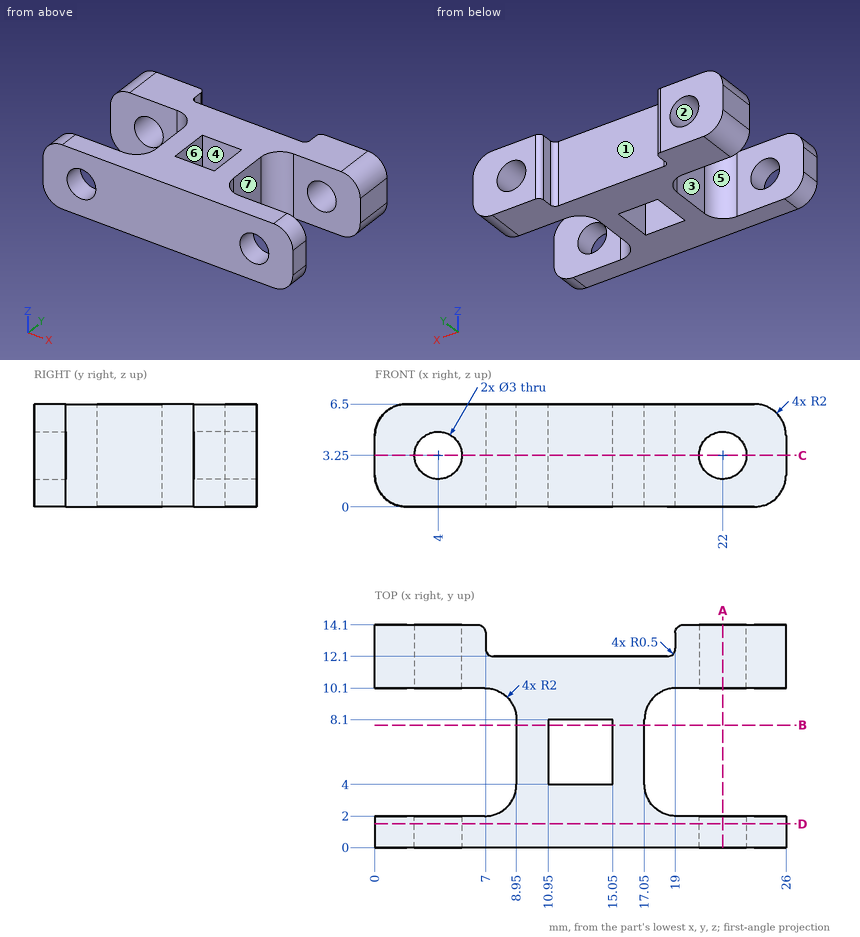
Drawing for the job (mm, zero at the part's lowest x, y, z). A direction names the side the tool comes from. Round coordinates to 2 decimals unless told otherwise and drop trailing zeros. Loops run counter-clockwise (first coordinate to the right, second up) from the corner with the lowest first, then second, coordinate; pieces in that order, holes last. Notation, with made-up numbers: (-7, 89) -> (1, 89) arc R16 ccw to (1, 113) -> close; hole circle Ø5 at (61.25, 64). An arc over 180 degrees is marked (long way). Use one line per item in the form item = value. Start each with the question number.
Item 1: Tool access for the marked faces 5, 6 and 7: list every direction of +Z, -Z, +X, -X, +Y, -Y with a clear straight run to the whole face (end or side of a thin tool).
Item 2: Band-saw the part on D-D (y = 1.5). List the corners of the cut face in (x, z).
Item 3: Two-plate mould, pull along Y, no slides. Class the marked faces 1, 2, 3 and 4: released by +Y, released by -Y, zero draft, split by the parting line, or undercut.
Item 4: Drill centre lines: line 1 along X through (y, z) = (11.1, 3.25); line 2 along Z through (x, y) = (22, 1.5); line 3 along Y through (x, z) = (13, 3.75). Where is each one in solid material? Low to high.
Item 5: Band-saw the part on C-C (z = 3.25). Give the number of separate pieces and of enclosed holes in the cut face, plus the area to 3 significant figures.
Item 6: Band-saw the part on B-B (y = 7.75). List the corners of the cut face in (x, z), plus the area to 3 significant figures.
Item 7: Band-saw the part on A-A (x = 22). List the corners of the cut face in (y, z), plus the area to 3 significant figures.
Item 8: Drop flat-ended pins along their axis: pin 1 Ø1.2 at (x, z) = (12, 3.5) entering from +Y; pin 2 Ø3.5 at (y, z) = (6.5, 2.5) entering from +X; pin 3 Ø3.5 at (y, z) = (7, 3) entering from -X. Give the stop position or say it passes through.
Data:
q1.face_5 = +Z, -Z, -X
q1.face_6 = +Z, -Z
q1.face_7 = +Z, -Z, +X
q2.outline = (0, 2) arc R2 ccw to (2, 0) -> (24, 0) arc R2 ccw to (26, 2) -> (26, 4.5) arc R2 ccw to (24, 6.5) -> (2, 6.5) arc R2 ccw to (0, 4.5) -> close; hole circle Ø3 at (4, 3.25); hole circle Ø3 at (22, 3.25)
q3.face_1 = released by +Y
q3.face_2 = zero draft
q3.face_3 = undercut
q3.face_4 = undercut
q4.line_1 = 0 to 2.5, 5.5 to 20.5, 23.5 to 26
q4.line_2 = 0 to 1.75, 4.75 to 6.5
q4.line_3 = 0 to 4, 8.1 to 12.1
q5.separate_pieces = 5
q5.enclosed_holes = 1
q5.area = 148 mm^2
q6.outline = (8.95, 0) -> (10.95, 0) -> (10.95, 6.5) -> (8.95, 6.5) -> close; (15.05, 0) -> (17.05, 0) -> (17.05, 6.5) -> (15.05, 6.5) -> close
q6.area = 26.0 mm^2
q7.outline = (0, 0) -> (2, 0) -> (2, 1.75) -> (0, 1.75) -> close; (0, 4.75) -> (2, 4.75) -> (2, 6.5) -> (0, 6.5) -> close; (10.1, 0) -> (14.1, 0) -> (14.1, 1.75) -> (10.1, 1.75) -> close; (10.1, 4.75) -> (14.1, 4.75) -> (14.1, 6.5) -> (10.1, 6.5) -> close
q7.area = 21.0 mm^2
q8.pin_1 = 12.1
q8.pin_2 = 17.06
q8.pin_3 = 8.84
